CAD build for the part. Positions are in the model's coordinates, mm. Face numbers are marked on the shaded views. A direction names the side the tool comes from. Round coordinates to 2 decimals unless told otherwise and drop trailing zeros. Order: outer loops, then holes, each group sorted by start corner. A loop starts at its lowest first (then second) coordinate and runs counter-clockwise, first axis right, second up. Notation, with made-up numbers: (42, 3) - (100, 3) arc R25 cw to (100, 25) - close; hole circle Ø6 at (89.5, 43). An arc over 180 degrees is marked (long way). Write item = value, one per line.
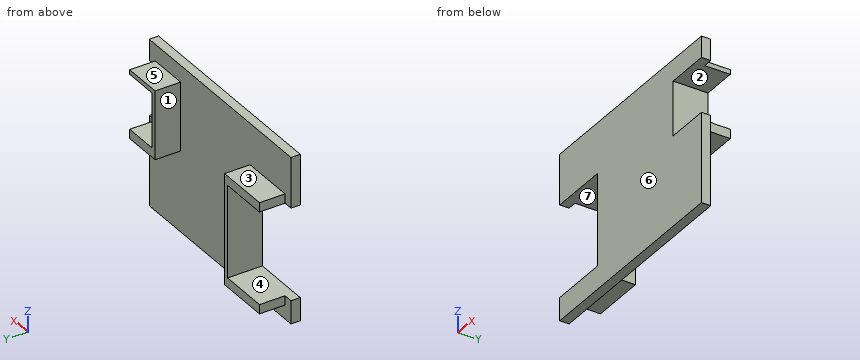
from build123d import *

# Parameters (mm, degrees)
ESQUISSE1_W             = 47.5
ESQUISSE1_H             = 35.8
BOSS_EXTRU_1_DEPTH      = 2
ESQUISSE2_W             = 9.5
ESQUISSE2_H             = 11.8
ENL_V_MAT_EXTRU_1_DEPTH = 10
ESQUISSE3_W             = 12.7
ESQUISSE3_H             = 19.9
ENL_V_MAT_EXTRU_2_DEPTH = 10
ESQUISSE5_W             = 1
ESQUISSE5_H             = 11.8
BOSS_EXTRU_2_DEPTH      = 5.5
ESQUISSE6_W             = 8.5
ESQUISSE6_H             = 1
BOSS_EXTRU_3_DEPTH      = 5.5
ESQUISSE7_W             = 8.5
ESQUISSE7_H             = 2
BOSS_EXTRU_4_DEPTH      = 5.5
ESQUISSE8_W             = 10.7
ESQUISSE8_H             = 2
BOSS_EXTRU_5_DEPTH      = 5.5
ESQUISSE9_W             = 1
ESQUISSE9_H             = 21.9
BOSS_EXTRU_6_DEPTH      = 5.5
ESQUISSE11_W            = 11.7
ESQUISSE11_H            = 2
BOSS_EXTRU_7_DEPTH      = 5.5


with BuildPart() as part:
    # Esquisse1 → Boss.-Extru.1 (new body)
    with BuildSketch(Plane(origin=(0, 0, 0), x_dir=(1, 0, 0), z_dir=(0, 1, 0))):
        with Locations((23.75, 17.9)):
            Rectangle(ESQUISSE1_W, ESQUISSE1_H)
    extrude(amount=BOSS_EXTRU_1_DEPTH)

    # Esquisse2 → Enlèv. mat.-Extru.1 (cut)
    with BuildSketch(Plane(origin=(0, 2, 0), x_dir=(1, 0, 0), z_dir=(0, 1, 0))):
        with Locations((42.75, 10.5)):
            Rectangle(ESQUISSE2_W, ESQUISSE2_H)
    extrude(amount=-ENL_V_MAT_EXTRU_1_DEPTH, mode=Mode.SUBTRACT)

    # Esquisse3 → Enlèv. mat.-Extru.2 (cut)
    with BuildSketch(Plane(origin=(0, 2, 0), x_dir=(1, 0, 0), z_dir=(0, 1, 0))):
        with Locations((6.35, 20.85)):
            Rectangle(ESQUISSE3_W, ESQUISSE3_H)
    extrude(amount=-ENL_V_MAT_EXTRU_2_DEPTH, mode=Mode.SUBTRACT)

    # Esquisse5 → Boss.-Extru.2 (add)
    with BuildSketch(Plane(origin=(0, 2, 0), x_dir=(1, 0, 0), z_dir=(0, 1, 0))):
        with Locations((37.5, 10.5)):
            Rectangle(ESQUISSE5_W, ESQUISSE5_H)
    extrude(amount=BOSS_EXTRU_2_DEPTH)

    # Esquisse6 → Boss.-Extru.3 (add)
    with BuildSketch(Plane(origin=(0, 2, 0), x_dir=(1, 0, 0), z_dir=(0, 1, 0))):
        with Locations((41.25, 4.1)):
            Rectangle(ESQUISSE6_W, ESQUISSE6_H)
    extrude(amount=BOSS_EXTRU_3_DEPTH)

    # Esquisse7 → Boss.-Extru.4 (add)
    with BuildSketch(Plane(origin=(0, 2, 0), x_dir=(1, 0, 0), z_dir=(0, 1, 0))):
        with Locations((41.25, 17.4)):
            Rectangle(ESQUISSE7_W, ESQUISSE7_H)
    extrude(amount=BOSS_EXTRU_4_DEPTH)

    # Esquisse8 → Boss.-Extru.5 (add)
    with BuildSketch(Plane(origin=(0, 2, 0), x_dir=(1, 0, 0), z_dir=(0, 1, 0))):
        with Locations((7.35, 31.8)):
            Rectangle(ESQUISSE8_W, ESQUISSE8_H)
    extrude(amount=BOSS_EXTRU_5_DEPTH)

    # Esquisse9 → Boss.-Extru.6 (add)
    with BuildSketch(Plane(origin=(0, 2, 0), x_dir=(1, 0, 0), z_dir=(0, 1, 0))):
        with Locations((13.2, 21.85)):
            Rectangle(ESQUISSE9_W, ESQUISSE9_H)
    extrude(amount=BOSS_EXTRU_6_DEPTH)

    # Esquisse11 → Boss.-Extru.7 (add)
    with BuildSketch(Plane(origin=(0, 2, 0), x_dir=(1, 0, 0), z_dir=(0, 1, 0))):
        with Locations((7.85, 9.9)):
            Rectangle(ESQUISSE11_W, ESQUISSE11_H)
    extrude(amount=BOSS_EXTRU_7_DEPTH)


solid = part.part
(1) Band-saw the part on B-B on x = 7. List the corners of the cut face in (y, z), plus the area to 3 significant figures.
Solved:
outline = (0, -35.8) - (2, -35.8) - (2, -32.8) - (7.5, -32.8) - (7.5, -30.8) - (0, -30.8) - close; (0, -10.9) - (7.5, -10.9) - (7.5, -8.9) - (2, -8.9) - (2, 0) - (0, 0) - close
area = 53.8 mm²
(2) Band-saw the part on D-D on x = 40. List the corners of the cut face in (y, z).
Solved:
outline = (0, -35.8) - (2, -35.8) - (2, -18.4) - (7.5, -18.4) - (7.5, -16.4) - (0, -16.4) - close; (0, -4.6) - (7.5, -4.6) - (7.5, -3.6) - (2, -3.6) - (2, 0) - (0, 0) - close
(3) Band-saw the part on C-C on z = -32. List the corners of the cut face in (x, y).
Solved:
outline = (0, 0) - (47.5, 0) - (47.5, 2) - (13.7, 2) - (13.7, 7.5) - (2, 7.5) - (2, 2) - (0, 2) - close
(4) Tool access for the marked faces 1, 2, 3 and 4: list every direction of +Z, -Z, +X, -X, +Y, -Y with a clear straight run to the whole face (end or side of a thin tool).
Solved:
face_1 = +Z, -Z, +Y
face_2 = +X, +Y, -Y
face_3 = +Z, -X, +Y
face_4 = -X, +Y, -Y
(5) Drop flat-ended pins along their axis: pin 1 (1.6 mm diameter, centred on y = 6, z = -17.5, fed in from +X); pin 2 (1 mm diameter, centred on y = 4.5, z = -30.5, fed in from +X); pin 3 (4 mm diameter, centred on y = 4.5, z = -8, fed in from +X); pin 4 (1.5 mm diameter, centred on x = 5.5, z = -13, fed in from +Y). Give the stop position or say it passes through.
Solved:
pin_1 = 45.5
pin_2 = 13.7
pin_3 = 38
pin_4 = through
(6) Band-saw the part on A-A on y = 5. List the corners of the cut face in (x, z).
Solved:
outline = (2, -32.8) - (13.7, -32.8) - (13.7, -8.9) - (2, -8.9) - (2, -10.9) - (12.7, -10.9) - (12.7, -30.8) - (2, -30.8) - close; (37, -18.4) - (45.5, -18.4) - (45.5, -16.4) - (38, -16.4) - (38, -4.6) - (45.5, -4.6) - (45.5, -3.6) - (37, -3.6) - close
(7) Probe line 1 along Z through (x, y) = (10, 3); line 2 along X through (y, z) = (5.5, -14); line 3 along X through (y, z) = (6.5, -10.5). List the from-to ranges inside material, lowest first.
Solved:
line_1 = -32.8 to -30.8, -10.9 to -8.9
line_2 = 12.7 to 13.7, 37 to 38
line_3 = 2 to 13.7, 37 to 38
(8) Pull direction Z, two halves, no side cores. Call the marked faces 5, 6 and 7: released by +Z, released by -Z, zero draft, split by the parting line, or undercut.
Solved:
face_5 = released by +Z
face_6 = zero draft
face_7 = undercut
